Design review of the part built by this model. Coordinates are the model's own, in mm. A direction names the side the tool comes from. Give positions to 0.01 mm unless a question says otherwise; leave off trailing zeros. Order: outer loops, then holes, each group sorted by start corner. A loop starts at its lowest first (then second) coordinate and runs counter-clockwise, first axis right, second up. Notation, with made-up numbers: (-17, 78) -> (37, 78) arc R8 cw to (37, 90) -> close; hole circle Ø4 at (74.5, 45). An arc over 180 degrees is marked (long way). One line per item, written item: value.
from build123d import *

# Parameters (mm, degrees)
F0_W      = 85
F0_H      = 85
F1_DEPTH  = 10.5
F2_R      = 5.5
F3_DEPTH  = 10.501
F5_DEPTH  = 5
F6_R      = 8
F7_DEPTH  = 5
F8_D      = 6
F10_DEPTH = 5
F11_R     = 3
F12_DEPTH = 25


with BuildPart() as f1:
    # F0 (on Top) → F1 (new body)
    with BuildSketch(Plane.XY):
        Rectangle(F0_W, F0_H)
    extrude(amount=F1_DEPTH)

    # F2 (on face) → F3 (cut, through all)
    with BuildSketch(Plane.XY.offset(10.5)):
        with Locations((0, 12.8)):
            Circle(F2_R)
        with Locations((0, -12.8)):
            Circle(F2_R)
    extrude(amount=-F3_DEPTH, mode=Mode.SUBTRACT)

    # F4 (on face) → F5 (cut)
    with BuildSketch(Plane.XY.offset(10.5)):
        with BuildLine():
            Line((-5.5, -23), (5.5, -23))
            ThreePointArc((5.5, -23), (6.914214, -22.414214), (7.5, -21))
            Line((7.5, -21), (7.5, 21))
            ThreePointArc((7.5, 21), (6.914214, 22.414214), (5.5, 23))
            Line((5.5, 23), (-5.5, 23))
            ThreePointArc((-5.5, 23), (-6.914214, 22.414214), (-7.5, 21))
            Line((-7.5, 21), (-7.5, -21))
            ThreePointArc((-7.5, -21), (-6.914214, -22.414214), (-5.5, -23))
        make_face()
    extrude(amount=-F5_DEPTH, mode=Mode.SUBTRACT)

    # F6 (on face) → F7 (cut)
    with BuildSketch(Plane.XY.offset(10.5)):
        with Locations((30, 30)):
            Circle(F6_R)
        with Locations((30, -30)):
            Circle(F6_R)
        with Locations((-30, -30)):
            Circle(F6_R)
        with Locations((-30, 30)):
            Circle(F6_R)
    extrude(amount=-F7_DEPTH, mode=Mode.SUBTRACT)

    # F8 (through all)
    with Locations(Plane.XY.offset(10.5)):
        with Locations((-30, -30), (30, -30), (30, 30), (-30, 30)):
            Hole(F8_D / 2)

    # F9 (on face) → F10 (cut)
    with BuildSketch(Plane(origin=(0, 0, 0), x_dir=(1, 0, 0), z_dir=(0, 0, -1))):
        with BuildLine():
            ThreePointArc((35, 3.5), (30, 8.5), (25, 3.5))
            Line((25, 3.5), (25, -3.5))
            ThreePointArc((25, -3.5), (30, -8.5), (35, -3.5))
            Line((35, -3.5), (35, 3.5))
        make_face()
        with BuildLine():
            ThreePointArc((3.5, 25), (8.5, 30), (3.5, 35))
            Line((3.5, 35), (-3.5, 35))
            ThreePointArc((-3.5, 35), (-8.5, 30), (-3.5, 25))
            Line((-3.5, 25), (3.5, 25))
        make_face()
        with BuildLine():
            ThreePointArc((-25, 3.5), (-30, 8.5), (-35, 3.5))
            Line((-35, 3.5), (-35, -3.5))
            ThreePointArc((-35, -3.5), (-30, -8.5), (-25, -3.5))
            Line((-25, -3.5), (-25, 3.5))
        make_face()
        with BuildLine():
            Line((-3.5, -35), (3.5, -35))
            ThreePointArc((3.5, -35), (8.5, -30), (3.5, -25))
            Line((3.5, -25), (-3.5, -25))
            ThreePointArc((-3.5, -25), (-8.5, -30), (-3.5, -35))
        make_face()
    extrude(amount=-F10_DEPTH, mode=Mode.SUBTRACT)

    # F11 (on face) → F12 (cut)
    with BuildSketch(Plane(origin=(0, 0, 0), x_dir=(1, 0, 0), z_dir=(0, 0, -1))):
        with Locations((0, 30)):
            Circle(F11_R)
        with Locations((0, -30)):
            Circle(F11_R)
        with Locations((30, 0)):
            Circle(F11_R)
        with Locations((-30, 0)):
            Circle(F11_R)
    extrude(amount=-F12_DEPTH, mode=Mode.SUBTRACT)


solid = f1.part
Item 1: Add section A-A on y = 0. Give the boundary of the cut face in (x, z).
Returned:
outline: (-42.5, 0) -> (-35, 0) -> (-35, 5) -> (-33, 5) -> (-33, 10.5) -> (-42.5, 10.5) -> close; (-27, 5) -> (-25, 5) -> (-25, 0) -> (25, 0) -> (25, 5) -> (27, 5) -> (27, 10.5) -> (7.5, 10.5) -> (7.5, 5.5) -> (-7.5, 5.5) -> (-7.5, 10.5) -> (-27, 10.5) -> close; (33, 5) -> (35, 5) -> (35, 0) -> (42.5, 0) -> (42.5, 10.5) -> (33, 10.5) -> close
Item 2: To check wall thickness, follow line 1 along X through (y, z) = (0, 7.1); line 2 along Y through (x, z) = (-30, 7); line 3 along X through (y, z) = (1, 3.25). State the ranges of each line that lie inside material, in increasing order. Write a range as from..to.
Returned:
line 1: -42.5..-33, -27..-7.5, 7.5..27, 33..42.5
line 2: -42.5..-38, -22..-3, 3..22, 38..42.5
line 3: -42.5..-35, -25..25, 35..42.5
Item 3: Draft analysis for pull direction Y (two halves, no side actions). For faces 1 (the flat face through (-1, 42.5, 5)), 2 (the cylindrical face through (-0.716, -7.347, 2.788)), state which applies: pulls with the +Y half, pulls with the -Y half, needs draft (parallel to the pull), parting line crosses it, or undercut.
Returned:
face 1: pulls with the +Y half
face 2: undercut
Item 4: Machinability: for faces 3 (the cylindrical face through (-0.65, 32.93, 7.71)), 4 (the flat face through (-30.1, 26.6, 5.5)), 5 (the flat face through (-25, 0, 2)), which of the approach directions +Z, -Z, +X, -X, +Y, -Y give a long, thin tool a straight path to every point of the face, cutting with its end or side? Answer none if there is none.
Returned:
face 3: +Z, -Z
face 4: +Z
face 5: -Z
Item 5: Add section B-B on x = 30. Give the boundary of the cut face in (y, z).
Returned:
outline: (-42.5, 0) -> (-33, 0) -> (-33, 5.5) -> (-38, 5.5) -> (-38, 10.5) -> (-42.5, 10.5) -> close; (-27, 0) -> (-8.5, 0) -> (-8.5, 5) -> (-3, 5) -> (-3, 10.5) -> (-22, 10.5) -> (-22, 5.5) -> (-27, 5.5) -> close; (3, 5) -> (8.5, 5) -> (8.5, 0) -> (27, 0) -> (27, 5.5) -> (22, 5.5) -> (22, 10.5) -> (3, 10.5) -> close; (33, 0) -> (42.5, 0) -> (42.5, 10.5) -> (38, 10.5) -> (38, 5.5) -> (33, 5.5) -> close
Item 6: Clearance check with flat-ended pins moving along their axes: P1, Ø14.5, axis at x = -30, y = -30, coming from the +Z side; P2, Ø5, axis at x = -1, y = -29, coming from the -Z side; P3, Ø5, axis at x = 30, y = 0, coming from the -Z side. State where each tip first meets the part, or that it passes through.
Returned:
P1: z = 5.5
P2: z = 5
P3: through
Item 7: Add section C-C on z = 9.25. Count the separate pieces of the cut face and the enclosed holes in it, plus the area to 3 significant figures.
Returned:
separate pieces: 1
enclosed holes: 9
area: 5,620 mm²
